```python
from build123d import *

# Parameters (mm, degrees)
SKETCH1_R           = 28
SKETCH1_R_2         = 11.5
BOSS_EXTRUDE1_DEPTH = 2
CUT_EXTRUDE1_DEPTH  = 3
CIRPATTERN1_COUNT   = 4


with BuildPart() as part:
    # Sketch1 → Boss-Extrude1 (new body)
    with BuildSketch(Plane(origin=(0, 0, 0), x_dir=(1, 0, 0), z_dir=(0, 1, 0))):
        Circle(SKETCH1_R)
        Circle(SKETCH1_R_2, mode=Mode.SUBTRACT)
    extrude(amount=BOSS_EXTRUDE1_DEPTH)

    # Sketch2 → Cut-Extrude1 (cut, through all)
    with BuildSketch(Plane(origin=(0, 2, 0), x_dir=(1, 0, 0), z_dir=(0, 1, 0))):
        with BuildLine():
            ThreePointArc((21.954229866, 7.990686188), (19.198547424, 9.275682014), (17.913551597, 6.519999571))
            ThreePointArc((17.913551597, 6.519999571), (18.773590541, 3.310290537), (19.063203436, 0))
            ThreePointArc((19.063203436, 0), (21.213203436, -2.15), (23.363203436, 0))
            ThreePointArc((23.363203436, 0), (23.008263879, 4.056977701), (21.954229866, 7.990686188))
        make_face()
    cut_extrude1 = extrude(amount=-CUT_EXTRUDE1_DEPTH, mode=Mode.SUBTRACT)

    # CirPattern1: Cut-Extrude1 ×4 about axis
    cirpattern1_axis = Axis((0, 0, 0), (0, 1, 0))
    for i in range(1, CIRPATTERN1_COUNT):
        add(cut_extrude1.rotate(cirpattern1_axis, i * 360 / CIRPATTERN1_COUNT), mode=Mode.SUBTRACT)


solid = part.part
```
Verification items for the finished model (mm, model axes). A direction names the side the tool comes from. Coordinates: 2 decimals unless noted, no trailing zeros. Write each loop counter-clockwise with the first axis right and the second up, starting at its lowest first coordinate (ties: lowest second). Pieces come first, ordered by that corner, then holes. Notation, with made-up numbers: M 81.25,-6 L 124.25,-6 A21 ccw 124.25,18 Z; hole C 8.5,52.5 d5. An arc over 180 degrees is marked long. Answer as a JSON object with one key per item and string values. Group by question number.
(1) Release check for a two-part mould opening along X. For faces 3 (the face through (21.17, 1.01, 2.15)), 4 (the face through (25.865, 0.986, 10.724)), 5 (the face through (0, 2, 12)) record: +X half, -X half, draft (parallel to the pull), parting line (faces both ways), or undercut.
(2) Gauge pin test, flat ends, axial feed: pin 1 (1 mm diameter, centred on x = -15.5, y = 0.5, fed in from +Z); pin 2 (1 mm diameter, centred on y = 1, z = 12.5, fed in from -X); pin 3 (20.5 mm diameter, centred on x = 0, z = 0, fed in from -Y). Record the tip position at first contact, or that the pin passes through.
(3) Material ranges on line 1 (Z direction, x = 5, y = 1.8); line 2 (X direction, y = 0.4, z = -1.5) (1 decimal); line 3 (X direction, y = 1.5, z = -8), recorded low to high.
(4) Cross-section at A-A, the plane y = 0.8. Record the cut outline in (x, z).
(5) Cross-section at C-C, the plane x = -3.5. Record the cut outline in (y, z).
(6) Tool access check on faces 1 (the face through (3.356, 1.014, 18.765)), 2 (the face through (0, 0, 12)). Record the directions out of +Z, -Z, +X, -X, +Y, -Y that give a thin tool (end or side, any length) a straight path to the whole face; none if there is none.
(7) Cross-section at B-B, the plane z = -5. Record the cut outline in (x, y).
(8) Cross-section at D-D, the plane z = -24. Record the cut outline in (x, y), and give its area (3 significant figures).
Reply:
{
 "1": {"face 3": "undercut", "face 4": "parting line", "face 5": "draft"},
 "2": {"pin 1": "z = 23.64", "pin 2": "x = -25.3", "pin 3": "through"},
 "3": {"line 1": "-27.55 to -10.36, 10.36 to 18.4, 22.82 to 27.55", "line 2": "-28 to -22.8, -19.7 to -11.4, 11.4 to 19, 23.3 to 28", "line 3": "-26.83 to -8.26, 8.26 to 17.92, 21.95 to 26.83"},
 "4": {"outline": "C 0,0 d56; hole M -23.36,0 A2.15 ccw -19.06,0 A19.06 cw -17.91,6.52 A2.15 ccw -21.95,7.99 A23.36 ccw Z; hole C 0,0 d23; hole M -7.99,-21.95 A23.36 ccw 0,-23.36 A2.15 ccw 0,-19.06 A19.06 cw -6.52,-17.91 A2.15 ccw Z; hole M 0,19.06 A19.06 cw 6.52,17.91 A2.15 ccw 7.99,21.95 A23.36 ccw 0,23.36 A2.15 ccw Z; hole M 17.91,-6.52 A2.15 ccw 21.95,-7.99 A23.36 ccw 23.36,0 A2.15 ccw 19.06,0 A19.06 cw Z"},
 "5": {"outline": "M 0,-27.78 L 2,-27.78 L 2,-23.1 L 0,-23.1 Z; M 0,-18.74 L 2,-18.74 L 2,-10.95 L 0,-10.95 Z; M 0,10.95 L 2,10.95 L 2,27.78 L 0,27.78 Z"},
 "6": {"face 1": "+Y, -Y", "face 2": "+Z, -Z, +X, -X, -Y"},
 "7": {"outline": "M -27.55,0 L -10.36,0 L -10.36,2 L -27.55,2 Z; M 10.36,0 L 18.4,0 L 18.4,2 L 10.36,2 Z; M 22.82,0 L 27.55,0 L 27.55,2 L 22.82,2 Z"},
 "8": {"outline": "M -14.42,0 L 14.42,0 L 14.42,2 L -14.42,2 Z", "area": "57.7 mm²"}
}
